The model under review builds one solid part; all positions refer to its coordinate system, in mm. A direction names the side the tool comes from. Coordinates: 2 decimals unless noted, no trailing zeros. Order: outer loops, then holes, each group sorted by start corner. A loop starts at its lowest first (then second) coordinate and runs counter-clockwise, first axis right, second up. Notation, with made-up numbers: M 35.25,9 L 92.25,9 A21 ccw 92.25,31 Z; hole C -26.5,48.5 d4. An arc over 180 degrees is marked long. Answer as CSV lines item,"result". Start each with the question number.
Q1. For P1, Ø6, axis at x = 23, y = 1, coming from the +Z side; P2, Ø1, axis at x = 24.5, y = -7.5, coming from the -Z side; P3, Ø4, axis at x = 29.5, z = -0.5, coming from the -Y side; P4, Ø8, axis at y = 4.5, z = 2.5, coming from the -X side, all flat-tipped, find the tip position at first contact; note any pin that passes through.
Q2. Consider section A-A on x = 48. Write out the cut boundary in (y, z) (1 decimal), and give its area (3 significant figures).
Q3. Wall thickness on L1, parallel to Z at x = 15, y = 0; L2, parallel to Z at x = 57, y = 0: over which ranges is each line inside the solid? List them lowest first. Write a range as [from, to].
Q4. The part is to be moulded in two halves that separate along Z. For faces 1 (the face through (34.925, -2, 8)), 2 (the face through (35.708, -7.559, 5.796)), 3 (the face through (23.88, 1.24, -6.78)), say which applies: +Z half, -Z half, draft (parallel to the pull), parting line (faces both ways), or undercut.
Q5. Machinability: for faces 4 (the face through (51.594, 3, 6)), 5 (the face through (11.178, -6.489, 2.314)), 6 (the face through (57.855, 3.219, -5.474)), 7 (the face through (3.41, -1.38, -6.2)), 8 (the face through (57.855, 3.131, 5.525)), which of the approach directions +Z, -Z, +X, -X, +Y, -Y give a long, thin tool a straight path to every point of the face, cutting with its end or side? Answer none if there is none.
Autodesk Inventor part; units mm, degrees
ref_plane "YZ Plane" through (0, 0, 0) normal (1, 0, 0) x (0, 1, 0)
ref_plane "XZ Plane" through (0, 0, 0) normal (0, 1, 0) x (-1, 0, 0)
ref_plane "XY Plane" through (0, 0, 0) normal (0, 0, 1) x (1, 0, 0)
sketch "Sketch1" plane through (0, 0, 0) normal (0, 0, 1) x (1, 0, 0)
  line L0 (0, 0) -> (8.7313, 0) construction
  line L1 (0, 0) -> (0, 6.35) construction
  line L2 (0, 7.9375) -> (8.7312, 7.9375)
  line L3 (8.7312, 7.9375) -> (8.7313, 0) construction
  line L4 (8.7312, 7.9375) -> (34.925, 7.9375)
  line L5 (8.7312, 7.9375) -> (8.7312, 14.2875) construction
  line L6 (8.7312, 14.2875) -> (9.525, 14.2875) construction
  line L7 (9.525, 14.2875) -> (9.525, 0) construction
  line L8 (9.525, 0) -> (8.7313, 0) construction
  line L9 (9.525, 0) -> (19.05, 0) construction
  line L10 (19.05, 0) -> (19.05, 26.67) construction
  line L11 (19.05, 26.67) -> (9.525, 26.67) construction
  line L12 (9.525, 26.67) -> (9.525, 14.2875) construction
  line L13 (14.2875, 0) -> (14.2875, 26.67) construction
  line L14 (14.2875, 17.4625) -> (21.4312, 17.4625) construction
  line L15 (21.4312, 17.4625) -> (21.4313, 0) construction
  line L16 (21.4313, 0) -> (19.05, 0) construction
  line L17 (21.4313, 0) -> (22.225, 0) construction
  line L18 (22.225, 0) -> (22.225, 14.2875) construction
  line L19 (22.225, 14.2875) -> (21.4313, 14.2875) construction
  line L20 (21.4313, 14.2875) -> (21.4313, 0) construction
  line L21 (22.225, 0) -> (31.75, 0) construction
  line L22 (31.75, 0) -> (31.75, 20.32) construction
  line L23 (31.75, 20.32) -> (22.225, 20.32) construction
  line L24 (22.225, 20.32) -> (22.225, 0) construction
  line L25 (26.9875, 20.32) -> (26.9875, 0) construction
  line L26 (26.9875, 17.4625) -> (34.1313, 17.4625) construction
  line L27 (34.1313, 17.4625) -> (34.1313, 0) construction
  line L28 (34.1313, 0) -> (31.75, 0) construction
  line L29 (34.1313, 0) -> (34.925, 0) construction
  line L30 (34.925, 0) -> (34.925, 14.2875) construction
  line L31 (34.925, 14.2875) -> (34.1313, 14.2875) construction
  line L32 (34.1313, 14.2875) -> (34.1313, 0) construction
  line L33 (34.925, 0) -> (36.5125, 0) construction
  line L34 (36.5125, 0) -> (36.5125, 7.9375) construction
  line L35 (36.5125, 9.525) -> (34.925, 9.525)
  line L36 (34.925, 9.525) -> (34.925, 7.9375)
  line L37 (45.2438, 7.9375) -> (45.2438, 0) construction
  line L38 (45.2438, 0) -> (36.5125, 0)
  line L39 (11.9063, 26.67) -> (11.9063, 0) construction
  line L40 (24.6063, 20.32) -> (24.6063, 0) construction
  line L41 (0, 7.9375) -> (0, 17.4625) construction
  line L42 (0, 17.4625) -> (8.7312, 17.4625) construction
  line L43 (8.7312, 17.4625) -> (8.7312, 14.2875) construction
  line L44 (0, 3.175) -> (45.2438, 3.175) construction
  circle A0 centre (11.9063, 5.5562) radius 2.3813 construction
  circle A1 centre (24.6063, 5.5562) radius 2.3812 construction
  circle A2 centre (11.9063, 5.8103) radius 2.3813 construction
  circle A3 centre (11.9063, 7.5565) radius 2.3813 construction
  circle A4 centre (24.6063, 5.8103) radius 2.3812 construction
  circle A5 centre (24.6063, 7.5565) radius 2.3812 construction
  line L45 (9.525, 8.1915) -> (14.2875, 8.1915) construction
  line L46 (12.6386, 3.175) -> (14.6388, 5.1753) construction
  line L47 (14.6388, 5.1753) -> (21.8737, 5.1753) construction
  line L48 (21.8737, 5.1753) -> (23.8739, 3.175) construction
  line L49 (22.225, 8.1915) -> (26.9875, 8.1915) construction
  line L50 (10.3187, 5.1753) -> (17.4901, 5.1753) construction
  line L51 (26.1938, 5.1753) -> (19.0224, 5.1753) construction
  line L52 (0, 6.35) -> (6.731, 6.35)
  line L53 (6.731, 6.35) -> (6.731, 5.5562)
  line L54 (10.3187, 5.1753) -> (8.3185, 3.175) construction
  line L55 (17.4901, 5.1753) -> (19.4903, 3.175) construction
  line L56 (19.4903, 3.175) -> (26.1938, 3.175) construction
  line L57 (26.1938, 3.175) -> (28.1015, 0) construction
  line L58 (26.1938, 5.1753) -> (28.194, 3.175) construction
  line L59 (28.194, 3.175) -> (34.8974, 3.175) construction
  line L60 (34.8974, 3.175) -> (36.8052, 0) construction
  line L61 (6.731, 5.5562) -> (33.8635, 5.5563)
  line L62 (37.202, 0) -> (33.8635, 5.5563)
  line L63 (19.0224, 5.1753) -> (17.0222, 3.175) construction
  line L64 (17.0222, 3.175) -> (-3.175, 3.175) construction
  line L65 (45.2438, 7.9375) -> (45.2438, 17.4625) construction
  line L66 (45.2438, 17.4625) -> (36.5125, 17.4625) construction
  line L67 (36.5125, 17.4625) -> (36.5125, 9.525) construction
  line L68 (45.2438, 7.9375) -> (51.5938, 7.9375)
  line L69 (51.5938, 7.9375) -> (51.5938, 0)
  line L70 (51.5938, 0) -> (45.2438, 0)
  line L71 (51.5938, 6.35) -> (64.2938, 6.35) construction
  line L72 (64.2938, 6.35) -> (64.2938, 0) construction
  line L73 (64.2938, 0) -> (51.5938, 0) construction
  line L74 (-8.1534, 3.175) -> (-8.1534, 2.3812) construction
  line L75 (-8.1534, 0) -> (36.8052, 0) construction
  line L76 (-3.175, 3.175) -> (-3.175, 2.3812) construction
  line L77 (-3.175, 2.3812) -> (-8.1534, 2.3812) construction
  line L78 (-8.1534, 3.175) -> (-8.1534, 6.35) construction
  line L79 (-8.1534, 6.35) -> (-3.175, 6.35) construction
  line L80 (-3.175, 6.35) -> (-3.175, 3.175) construction
  line L81 (-3.175, 0) -> (-3.175, 2.3812) construction
  line L82 (-0.7937, 0) -> (-0.7938, 11.1125) construction
  line L83 (-0.7938, 11.1125) -> (-3.175, 11.1125) construction
  line L84 (-3.175, 11.1125) -> (-3.175, 6.35) construction
  line L85 (-3.175, 3.175) -> (-8.1534, 3.175) construction
  line L86 (-8.1534, 2.3812) -> (-8.1534, 0) construction
  line L87 (-8.1534, 2.7051) -> (-9.652, 2.7051) construction
  line L88 (-9.652, 2.7051) -> (-9.652, 0) construction
  line L89 (-9.652, 0) -> (-8.1534, 0) construction
  line L90 (-8.1534, 1.4224) -> (-5.6134, 1.4224) construction
  line L91 (-5.6134, 1.4224) -> (-5.6134, 0) construction
  line L92 (-5.6134, 1.4224) -> (-3.0734, 1.4224) construction
  line L93 (-3.0734, 1.4224) -> (-3.0734, 0) construction
  line L94 (-3.175, 11.1125) -> (-13.4938, 11.1125) construction
  line L95 (-13.4938, 11.1125) -> (-13.4937, 5.9531) construction
  line L96 (-13.4937, 5.9531) -> (-18.5801, 5.9531) construction
  line L97 (-18.5801, 5.9531) -> (-18.5801, 0) construction
  line L98 (-18.5801, 0) -> (-9.652, 0) construction
  line L99 (-8.1534, 3.9687) -> (-14.6113, 3.9687) construction
  line L100 (-14.6113, 3.9687) -> (-14.6113, 0) construction
  line L101 (-14.6113, 3.429) -> (-10.4457, 3.429) construction
  line L102 (-10.4457, 3.429) -> (-10.4457, 0) construction
  line L103 (-16.9926, 3.175) -> (-16.9926, 0) construction
  line L104 (-16.9926, 3.175) -> (-18.5801, 3.175) construction
  line L105 (0, 6.35) -> (0, 7.9375)
  line L106 (6.731, 5.5562) -> (6.731, 0) construction
  line L107 (33.8635, 5.5563) -> (45.2438, 5.5563) construction
  line L108 (34.925, 7.9375) -> (34.925, 0) construction
  line L109 (36.5125, 7.9375) -> (36.5125, 9.525)
  line L110 (36.5125, 7.9375) -> (45.2438, 7.9375)
  line L111 (34.925, 7.9375) -> (36.5125, 7.9375) construction
  dimension "d1" = 7.9375
  dimension "d2" = 0.7937
  dimension "d3" = 14.2875
  dimension "d4" = 9.525
  dimension "d5" = 26.67
  dimension "d6" = 7.1437
  dimension "d7" = 17.4625
  dimension "d8" = 0.7937
  dimension "d9" = 14.2875
  dimension "d10" = 9.525
  dimension "d11" = 20.32
  dimension "d12" = 7.1437
  dimension "d13" = 17.4625
  dimension "d14" = 0.7937
  dimension "d15" = 14.2875
  dimension "d16" = 1.5875
  dimension "d17" = 9.525
  dimension "d18" = 8.7312
  dimension "d19" = 2.3813
  dimension "d20" = 2.3813
  dimension "d21" = 17.4625
  dimension "d22" = 3.175
  dimension "d23" = 4.7625
  dimension "d24" = 4.7625
  dimension "d26" = 0.254
  dimension "d28" = 45
  dimension "d29" = 45
  dimension "d30" = 0.254
  dimension "d31" = 7.2348
  dimension "d32" = 5.1753
  dimension "d33" = 7.1713
  dimension "d34" = 1.5875
  dimension "d35" = 7.1713
  dimension "d36" = 1.5875
  dimension "d37" = 6.35
  dimension "d39" = 45
  dimension "d40" = 45
  dimension "d41" = 1.5875
  dimension "d42" = 59
  dimension "d43" = 6.7034
  dimension "d44" = 6.7034
  dimension "d46" = 0.3969
  dimension "d52" = 17.4625
  dimension "d53" = 6.35
  dimension "d54" = 12.7
  dimension "d55" = 6.35
  dimension "d56" = 2.3813
  dimension "d57" = 4.9784
  dimension "d58" = 6.35
  dimension "d66" = 2.3813
  dimension "d67" = 0.7937
  dimension "d68" = 11.1125
  dimension "d69" = 2.7051
  dimension "d70" = 1.4986
  dimension "d71" = 1.4224
  dimension "d72" = 2.54
  dimension "d73" = 2.54
  dimension "d74" = 3.9688
  dimension "d75" = 4.1656
  dimension "d76" = 3.429
  dimension "d77" = 0.7937
  dimension "d78" = 3.175
  dimension "d79" = 2.3813
  dimension "d80" = 1.5875
revolve "Revolution1" add sketch "Sketch1" angle 360 about axis through (9.525, 0, 0) along (1, 0, 0)
sketch "Sketch2" plane through (51.5938, 0, 0) normal (1, 0, 0) x (0, 0, -1)
  circle A0 centre (0, 0) radius 7.9375
  line L0 (-7.3323, 0) -> (-3.6662, 6.35)
  line L1 (-3.6662, 6.35) -> (3.6662, 6.35)
  line L2 (3.6662, 6.35) -> (7.3323, 0)
  line L3 (7.3323, 0) -> (3.6662, -6.35)
  line L4 (3.6662, -6.35) -> (-3.6662, -6.35)
  line L5 (-3.6662, -6.35) -> (-7.3323, 0)
  dimension "d88" = 12.7
extrude "Extrusion1" add sketch "Sketch2" along normal blind 12.7 contours L0 L1 L2 L3 L4 L5
sketch "Sketch3" plane through (0, 0, 0) normal (0, 1, 0) x (-1, 0, 0)
  point P0 (0, 0)
  point P1 (-11.9063, 0)
  point P2 (-24.6063, 0)
hole "Hole1" at (11.9063, 0, 0) at (24.6063, 0, 0) direction (0, -1, 0) diameter 4.8514 end through all
pattern_circular "Circular Pattern1" count 3 over 360 about axis through (-10, 0, 0) along (1, 0, 0) of "Hole1"
ref_plane "Work Plane1" through (10.3187, 5.1753, 0) normal (-1, 0, 0) x (0, 0, 1)
ref_plane "Work Plane2" through (26.1938, 3.175, 0) normal (-1, 0, 0) x (0, 0, 1)
ref_plane "Work Plane3" through (17.4901, 5.1753, 0) normal (-1, 0, 0) x (0, 0, 1)
sketch "Sketch4" plane through (64.2938, 0, 0) normal (1, 0, 0) x (0, 0, -1)
  point P0 (0, 0)
  point P1 (0, 0)
hole "Hole2" at (64.2938, 0, 0) direction (-1, 0, 0) diameter 4.9784 depth 19.05 tip angle 118
equation "\"d9\" = d3"
equation "\"d12\" = d6"
equation "\"d13\" = d7"
equation "\"d15\" = d9"
equation "\"d18\" = d0"
equation "\"d20\" = d19"
equation "\"d35\" = d33"
equation "\"d36\" = d34"
equation "\"d43\" = d44"
equation "\"d52\" = d13"
properties part number "Ball Shifting Outline" material "Steel, Alloy"
Evaluation:
1,P1,"stops at z = 7.94"
1,P2,"stops at z = -3.74"
1,P3,"stops at y = -7.94"
1,P4,"stops at x = 0"
2,outline,"C 0,0 d15.9; hole C 0,0 d5"
2,area,"178 mm²"
3,L1,"z = [-7.94, -5.56], [5.56, 7.94]"
3,L2,"z = [-7.33, -2.49], [2.49, 7.33]"
4,face 1,"draft"
4,face 2,"parting line"
4,face 3,"undercut"
5,face 4,"+X"
5,face 5,"-Y"
5,face 6,"-Z, +X, +Y"
5,face 7,"-X"
5,face 8,"+Z, +X, +Y"
